Build history of the part. All positions in model axes, mm. A direction names the side the tool comes from. Coordinates: 2 decimals unless noted, no trailing zeros. Loops run counter-clockwise (first coordinate to the right, second up) from the corner with the lowest first, then second, coordinate; pieces in that order, holes last. Notation, with made-up numbers: (83, -9) - (87, -9) arc R8 cw to (87, -1) - close; hole circle Ø4 at (35, 47.25). An arc over 180 degrees is marked (long way). One line per item, written item: value.
```python
from build123d import *

# Parameters (mm, degrees)
EXTRUDE_THIN1_DEPTH                          = 502
SKETCH3_W                                    = 50
SKETCH3_H                                    = 30
BOSS_EXTRUDE1_DEPTH                          = 2
CSK_FOR_M3_COUNTERSUNK_FLAT_HEAD_SCR_2_COUNT = 2
CSK_FOR_M3_COUNTERSUNK_FLAT_HEAD_SCR_2_PITCH = 13


with BuildPart() as part:
    # Sketch1 → Extrude-Thin1 (new body)
    with BuildSketch(Plane.XY):
        with BuildLine():
            Line((94.25, -50), (75.246672681, -0.640708262))
            ThreePointArc((75.246672681, -0.640708262), (74.879445737, -0.175593626), (74.313447388, 0))
            Line((74.313447388, 0), (-74.313447388, 0))
            ThreePointArc((-74.313447388, 0), (-74.879445737, -0.175593626), (-75.246672681, -0.640708262))
            Line((-75.246672681, -0.640708262), (-94.25, -50))
            Line((-94.25, -50), (-96.116450586, -49.281416525))
            Line((-96.116450586, -49.281416525), (-77.113123267, 0.077875213))
            ThreePointArc((-77.113123267, 0.077875213), (-76.011442435, 1.473219121), (-74.313447388, 2))
            Line((-74.313447388, 2), (74.313447388, 2))
            ThreePointArc((74.313447388, 2), (76.011442435, 1.473219121), (77.113123267, 0.077875213))
            Line((77.113123267, 0.077875213), (96.116450586, -49.281416525))
            Line((96.116450586, -49.281416525), (94.25, -50))
        make_face()
    extrude(amount=EXTRUDE_THIN1_DEPTH)

    # Sketch3 → Boss-Extrude1 (add)
    with BuildSketch(Plane.XY.offset(502)):
        with Locations((0, 15)):
            Rectangle(SKETCH3_W, SKETCH3_H)
        with BuildLine():
            Line((2, 22), (2, 8))
            ThreePointArc((2, 8), (0, 6), (-2, 8))
            Line((-2, 8), (-2, 22))
            ThreePointArc((-2, 22), (0, 24), (2, 22))
        make_face(mode=Mode.SUBTRACT)
    extrude(amount=-BOSS_EXTRUDE1_DEPTH)

    # Mirror1: part across plane


with BuildPart() as part_1:
    add(part.part)
    add(part.part.mirror(Plane.XY.offset(251)))

    # Sketch5 → CSK for M3 Countersunk Flat Head Screw1 (revolve, cut)
    with BuildSketch(Plane(origin=(0, 2, 19), x_dir=(0, 0, 1), z_dir=(1, 0, 0))):
        Polygon((0, 0), (0, 26.021463052), (1.7, 25), (1.7, 1.45), (3.15, 0), align=None)
    csk_for_m3_countersunk_flat_head_screw1 = revolve(axis=Axis((0, 8.35, 19), (0, -1, 0)), mode=Mode.SUBTRACT)

    # CSK for M3 Countersunk Flat Head Scr 2: CSK for M3 Countersunk Flat Head Screw1 ×2
    with Locations(*[(0, 0, -i * CSK_FOR_M3_COUNTERSUNK_FLAT_HEAD_SCR_2_PITCH) for i in range(1, CSK_FOR_M3_COUNTERSUNK_FLAT_HEAD_SCR_2_COUNT)]):
        add(csk_for_m3_countersunk_flat_head_screw1, mode=Mode.SUBTRACT)

    # Mirror2: CSK for M3 Countersunk Flat Head Screw1 across plane
    add(csk_for_m3_countersunk_flat_head_screw1.mirror(Plane.XY.offset(251)), mode=Mode.SUBTRACT)

    # Mirror2 copy 1 sketch → Mirror2 copy 1 (revolve, cut)
    with BuildSketch(Plane(origin=(0, 2, 496), x_dir=(0, 0, -1), z_dir=(1, 0, 0))):
        Polygon((0, 0), (0, -26.021463052), (1.7, -25), (1.7, -1.45), (3.15, 0), align=None)
    revolve(axis=Axis((0, 8.35, 496), (0, 1, 0)), mode=Mode.SUBTRACT)


solid = part_1.part
```
Item 1: Pull direction Z, two halves, no side cores. Call faces 1 (the face through (-1, 2, 247)), 2 (the face through (0, 5, 502)), 3 (the face through (-84.615, -24.975, 247.486)): released by +Z, released by -Z, zero draft, split by the parting line, or undercut.
Check result:
face 1: undercut
face 2: released by +Z
face 3: zero draft
Item 2: Tool access for faces 4 (the face through (-1, 0, 255)), 5 (the face through (86.5, -24.3, 247.5)), 6 (the face through (-6, 16, 500)): list every direction of +Z, -Z, +X, -X, +Y, -Y with a clear straight run to the whole face (end or side of a thin tool).
Check result:
face 4: +Z, -Z, -Y
face 5: +Z, -Z, +X, +Y
face 6: +X, -X, +Y
Item 3: Cut at B-B, the plane y = -11.5. Write the cut outline in (x, z), then the cut area to 3 significant figures.
Check result:
outline: (-81.57, 0) - (-79.43, 0) - (-79.43, 502) - (-81.57, 502) - close; (79.43, 0) - (81.57, 0) - (81.57, 502) - (79.43, 502) - close
area: 2,150 mm^2
Item 4: Cut at A-A, the plane y = 17. Write the cut outline in (x, z), then the cut area to 3 significant figures.
Check result:
outline: (-25, 0) - (-2, 0) - (-2, 2) - (-25, 2) - close; (-25, 500) - (-2, 500) - (-2, 502) - (-25, 502) - close; (2, 0) - (25, 0) - (25, 2) - (2, 2) - close; (2, 500) - (25, 500) - (25, 502) - (2, 502) - close
area: 184 mm^2
Item 5: Probe probe 1 along Z at (x, y) = (0, 0.3); probe 2 along Z at (x, y) = (8, 14); probe 3 along X at (y, z) = (0.25, 496). List the from-to ranges inside material, lowest first. Write a range as from..to.
Check result:
probe 1: z = 0..4.3, 7.7..17.3, 20.7..481.3, 484.7..494.3, 497.7..502
probe 2: z = 0..2, 500..502
probe 3: x = -77.04..-1.7, 1.7..77.04
Item 6: Drop flat-ended pins along their axis: P1, Ø2, axis at y = 13, z = 501, coming from the -X side; P2, Ø8, axis at x = 52.5, z = 428, coming from the -Y side; P3, Ø1.6, axis at y = 12.5, z = 501, coming from the +X side. Give the stop position or say it passes through.
Check result:
P1: stops at x = -25
P2: stops at y = 0
P3: stops at x = 25
Item 7: Cut at C-C, the plane z = 236. Write the cut outline in (x, y), then the cut area to 3 significant figures.
Check result:
outline: (-96.12, -49.28) - (-94.25, -50) - (-75.25, -0.64) arc R1 cw to (-74.31, 0) - (74.31, 0) arc R1 cw to (75.25, -0.64) - (94.25, -50) - (96.12, -49.28) - (77.11, 0.08) arc R3 ccw to (74.31, 2) - (-74.31, 2) arc R3 ccw to (-77.11, 0.08) - close
area: 518 mm^2
Item 8: Cut at D-D, the plane x = -41. Write the cut outline in (y, z).
Check result:
outline: (0, 0) - (2, 0) - (2, 502) - (0, 502) - close
